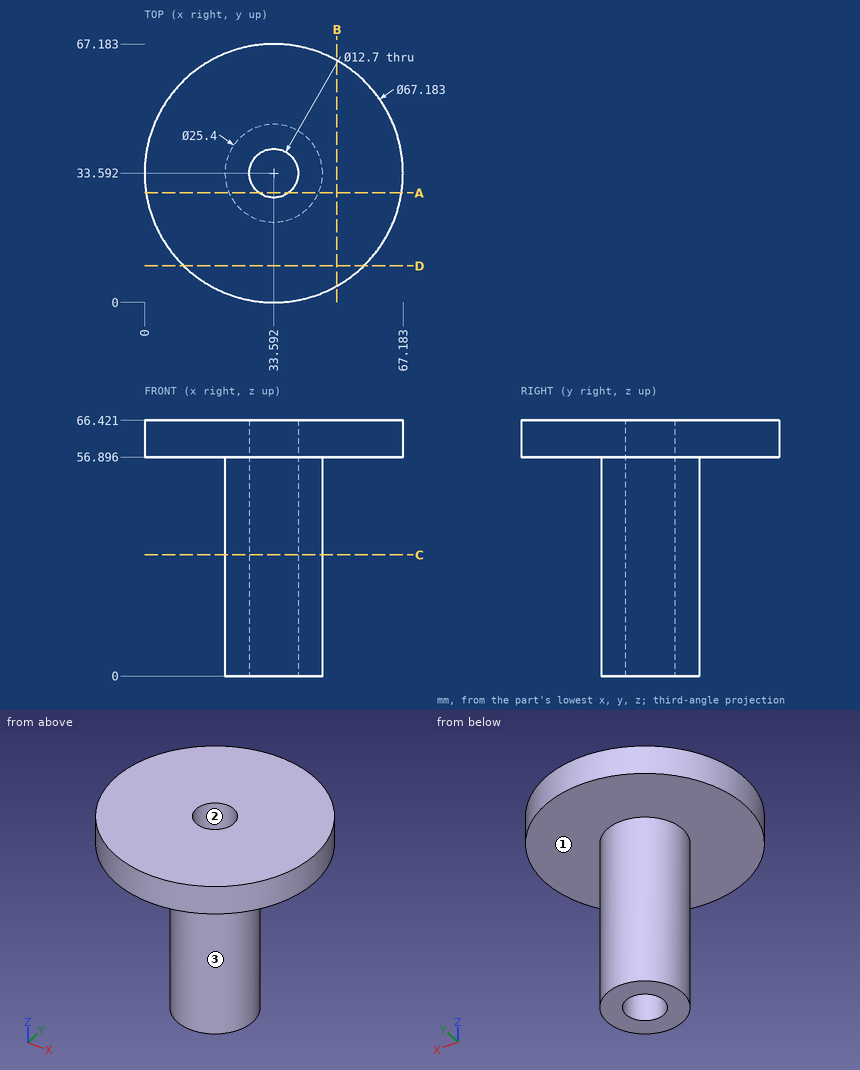
Job drawing, mm, ordinate dimensions from the low corner. One solid piece. Give positions to 0.01 mm unless a question says otherwise; leave off trailing zeros. Loops run counter-clockwise (first coordinate to the right, second up) from the corner with the lowest first, then second, coordinate; pieces in that order, holes last. Notation, with made-up numbers: (-10.75, -14) -> (10.25, -14) arc R29 ccw to (10.25, 7) -> close; hole circle Ø1 at (58.25, -14.75). An arc over 180 degrees is marked (long way). Write each question's results on one line, items separated by ' | '. Start each with the question number.
Q1. Band-saw the part on B-B on x = 50. List the corners of the cut face in (y, z) (1 decimal).
Q2. Pull direction X, two halves, no side cores. Call the marked faces 1, 2 and 3: +X half, -X half, draft (parallel to the pull), parting line (faces both ways), or undercut.
Q3. Band-saw the part on C-C on z = 31.5. List the corners of the cut face in (x, y), plus the area to 3 significant figures.
Q4. Band-saw the part on D-D on y = 9.5. List the corners of the cut face in (x, z) (1 decimal), plus the area to 3 significant figures.
Q5. Pin check, flat tips, straight feed: P1, Ø1, axis at y = 37, z = 8.5, coming from the -X side; P2, Ø5, axis at x = 46.5, z = 30.5, coming from the -Y side (1 decimal); P3, Ø10, axis at x = 14.5, z = 38, coming from the +Y side; P4, Ø4, axis at x = 7, y = 56.5, coming from the -Z side. Stop position of each tip, or through.
Q6. Band-saw the part on A-A on y = 28.5. List the corners of the cut face in (x, z) (1 decimal).
Q7. Wall check: L1, parallel to Z at x = 48, y = 49 (1 decimal); L2, parallel to Y at x = 36.5, z = 14 (1 decimal); L3, parallel to Y at x = 30, z = 49 (1 decimal). Give the ranges that are in metal, low to high.
Results are:
1) outline: (4.3, 56.9) -> (62.9, 56.9) -> (62.9, 66.4) -> (4.3, 66.4) -> close
2) face 1: draft | face 2: undercut | face 3: parting line
3) outline: circle Ø25.4 at (33.59, 33.59); hole circle Ø12.7 at (33.59, 33.59) | area: 380 mm²
4) outline: (10.2, 56.9) -> (57, 56.9) -> (57, 66.4) -> (10.2, 66.4) -> close | area: 446 mm²
5) P1: stops at x = 21.23 | P2: stops at y = 26.3 | P3: passes through | P4: stops at z = 56.9
6) outline: (0.4, 56.9) -> (22, 56.9) -> (22, 0) -> (29.8, 0) -> (29.8, 66.4) -> (0.4, 66.4) -> close; (37.4, 0) -> (45.2, 0) -> (45.2, 56.9) -> (66.8, 56.9) -> (66.8, 66.4) -> (37.4, 66.4) -> close
7) L1: z = 56.9 to 66.4 | L2: y = 21.2 to 27.9, 39.2 to 46 | L3: y = 21.4 to 28.4, 38.8 to 45.8
